from build123d import *

# Parameters (mm, degrees)
BOSS_EXTRUDE1_DEPTH  = 1.5875
M4_CLEARANCE_HOLE1_D = 4.5
SKETCH5_R            = 3
CUT_EXTRUDE1_DEPTH   = 4.1750001


with BuildPart() as part:
    # Sketch1 → Boss-Extrude1 (new body, symmetric)
    with BuildSketch(Plane.XY):
        with BuildLine():
            ThreePointArc((-35.147058824, -14.411764706), (-41.911764706, -12.352941176), (-39.852941176, -5.588235294))
            add(Edge.make_bspline(
                [(-39.852941176, -5.588235294), (-25.087835375, 2.313761515), (0, 5.671559621), (25.087835375, 2.313761515), (39.852941176, -5.588235294)],
                knots=[0, 0, 0, 0.375, 0.625, 1, 1, 1], degree=2))
            ThreePointArc((39.852941176, -5.588235294), (41.911764706, -12.352941176), (35.147058824, -14.411764706))
            add(Edge.make_bspline(
                [(-35.147058824, -14.411764706), (-21.787164625, -7.313761515), (0, -4.421559621), (21.787164625, -7.313761515), (35.147058824, -14.411764706)],
                knots=[0, 0, 0, 0.375, 0.625, 1, 1, 1], degree=2))
        make_face()
    extrude(amount=BOSS_EXTRUDE1_DEPTH, both=True)

    # M4 Clearance Hole1 (through all)
    with Locations(Plane.XY.offset(1.5875)):
        with Locations((37.5, -10), (-12.5, -1.111111111), (12.5, -1.111111111)):
            Hole(M4_CLEARANCE_HOLE1_D / 2)

    # Sketch5 → Cut-Extrude1 (cut, through all)
    with BuildSketch(Plane.XY.offset(1.5875)):
        with Locations((-37.5, -10)):
            Circle(SKETCH5_R)
    extrude(amount=-CUT_EXTRUDE1_DEPTH, mode=Mode.SUBTRACT)


solid = part.part
Design review of the part built by this model. Coordinates are the model's own, in mm. Coordinates: 2 decimals unless noted, no trailing zeros. One line per item, written item: value.
1) Draft analysis for pull direction Y (two halves, no side actions). For faces 1 (the face through (41.96, -12.26, 0.02)), 2 (the face through (36.29, -8.103, -0.022)), 3 (the face through (1, -2, 1.588)), state which applies: +Y half, -Y half, draft (parallel to the pull), parting line (faces both ways), or undercut.
Output values:
face 1: parting line
face 2: undercut
face 3: draft
2) We need section A-A, the plane y = -8.5. Count the separate pieces of the cut face and the enclosed holes in it, then the cut area to 3 significant figures.
Output values:
separate pieces: 4
enclosed holes: 0
area: 105 mm2
3) Clearance check with flat-ended pins moving along their axes: P1, Ø1.5, axis at x = 26, z = 0.5, coming from the -Y side; P2, Ø1, axis at x = -8.5, z = 0.5, coming from the -Y side; P3, Ø5, axis at x = -37.5, y = -10, coming from the -Z side. State where each tip first meets the part, or that it passes through.
Output values:
P1: stops at y = -10.47
P2: stops at y = -5.62
P3: passes through
4) To check wall thickness, follow probe 1 along X at (y, z) = (-12, -0.05); probe 2 along X at (y, z) = (-1.25, -0.7); probe 3 along Y at (x, z) = (12.5, -0.1). State the ranges of each line that lie inside material, in increasing order. Write a range as [from, to].
Output values:
probe 1: x = [-42.08, -39.74], [-35.26, -30.28], [30.28, 36.47], [38.53, 42.08]
probe 2: x = [-30.66, -14.75], [-10.25, 10.25], [14.75, 30.66]
probe 3: y = [-6.19, -3.36], [1.14, 3.96]
